Source: CAD feature listing. Evaluate the final solid. Frame: model axes, mm. A direction names the side the tool comes from. Give positions to 0.01 mm unless a question says otherwise; leave off trailing zeros. Write each loop counter-clockwise with the first axis right and the second up, starting at its lowest first coordinate (ties: lowest second). Pieces come first, ordered by that corner, then holes. Notation, with made-up numbers: (79.25, -14.75) -> (112.25, -14.75) arc R15 cw to (112.25, 9.25) -> close; hole circle Ø5 at (47, -24). An arc over 180 degrees is marked (long way). Answer as a JSON object with one key per item and string values. Group by question number.
Item 1: Section query A-A on z = 31. Return the cut outline in (x, y), plus the area to 3 significant figures.
Item 2: Pull-direction query (Y, two-part tool) for faces 1 (the face through (0, 30, 2)), 2 (the face through (0, 0, -19)), 3 (the face through (0, -30, 2)), 4 (the face through (26.438, 24.252, 1.726)); classes: pulls with the +Y half, pulls with the -Y half, needs draft (parallel to the pull), parting line crosses it, or undercut.
Item 3: Access query for faces 5 (the face through (0, -3, -13)), 6 (the face through (-23, -23, 3.5)), 7 (the face through (-1.615, 3.105, -9.367)), 8 (the face through (23, 23, 3.5)), 9 (the face through (-23, 23, 3.5)). Directions: +Z, -Z, +X, -X, +Y, -Y. A direction counts if a zero-diameter tool reaches every point of the face in a straight line with its end or side. Return the directions, or none.
Item 4: First-contact query: pin 1 Ø4 at (x, z) = (-1, -13.5) entering from -Y; pin 2 Ø1 at (x, z) = (0.5, -7) entering from +Y; pin 3 Ø3.5 at (x, y) = (25, 25) entering from -Z. Flat tips, straight axial feed; report the tip coordinate or a pass-through.
Item 5: Ray query, probe 1 along X at (y, z) = (25, 2); probe 2 along Z at (x, y) = (-7, -7.5). Return the intervals inside material, ascending. Write a range as from..to.
Autodesk Inventor part; units mm, degrees
ref_plane "YZ Plane" through (0, 0, 0) normal (1, 0, 0) x (0, 1, 0)
ref_plane "XZ Plane" through (0, 0, 0) normal (0, 1, 0) x (-1, 0, 0)
ref_plane "XY Plane" through (0, 0, 0) normal (0, 0, 1) x (1, 0, 0)
sketch "Esquisse1" plane through (0, 0, 0) normal (0, 0, 1) x (1, 0, 0)
  line L0 (-25.5, -30) -> (25.5, -30)
  line L1 (30, -25.5) -> (30, 25.5)
  line L2 (25.5, 30) -> (-25.5, 30)
  line L3 (-30, 25.5) -> (-30, -25.5)
  line L4 (-30, -30) -> (30, 30) construction
  line L5 (30, -30) -> (-30, 30) construction
  arc A0 (-30, -25.5) -> (-25.5, -30) centre (-25.5, -25.5) ccw
  arc A1 (25.5, -30) -> (30, -25.5) centre (25.5, -25.5) ccw
  arc A2 (30, 25.5) -> (25.5, 30) centre (25.5, 25.5) ccw
  arc A3 (-25.5, 30) -> (-30, 25.5) centre (-25.5, 25.5) ccw
  point P0 (0, 0)
  dimension "d0" = 60
  dimension "d1" = 60
  dimension "d2" = 4.5
extrude "Embase" add sketch "Esquisse1" along normal blind 3.5
sketch "Esquisse3" plane through (0, 0, 3.5) normal (0, 0, 1) x (1, 0, 0)
  point P0 (0, 0)
  point P1 (-25, -25)
  point P2 (-25, 25)
  point P3 (25, 25)
  point P4 (25, -25)
  dimension "Entraxe_moteur" = 50
  dimension "d8" = 50
  dimension "d9" = 25
  dimension "d10" = 25
hole "Perçage1" at (-25, -25, 3.5) at (-25, 25, 3.5) at (25, 25, 3.5) at (25, -25, 3.5) direction (0, 0, -1) diameter 3.242 end through all
sketch "Esquisse2" plane through (0, 0, 3.5) normal (0, 0, 1) x (1, 0, 0)
  circle A0 centre (0, 0) radius 30
  line L0 (-30, 25.5) -> (-30, -25.5)
extrude "Extrusion2" add sketch "Esquisse2" along normal blind 59
fillet "Congé1" radius 3 1 edges at (-30, 0, 62.5)
sketch "Esquisse4" plane through (0, 0, 0) normal (0, 0, -1) x (-1, 0, 0)
  circle A0 centre (0, 0) radius 3.5
  dimension "d19" = 7
extrude "Extrusion3" add sketch "Esquisse4" along normal blind 19
sketch "Esquisse5" plane through (0, 0, -19) normal (0, 0, -1) x (-1, 0, 0)
  line L0 (-1.8028, -3) -> (1.8028, -3)
  circle A0 centre (0, 0) radius 3.5
  dimension "d22" = 6.5
extrude "Extrusion4" cut sketch "Esquisse5" against normal blind 15 contours L0 A0 picked at (0.3722, -3.1057)
sketch "Esquisse6" plane through (-1.8028, -3, -19) normal (0, -1, 0) x (1, 0, 0)
  line L0 (3.6056, 0) -> (0, 0)
  point P0 (1.8028, 19)
  point P1 (1.8028, 8)
  point P2 (1.8028, 0)
  dimension "d25" = 8
hole "Perçage2" at (0, -3, -11) direction (0, 1, 0) diameter 3.4 end through all
properties part number "Moteur" material "Acier inoxydable"
Worked answers:
{
 "1": {"outline": "circle Ø60 at (0, 0)", "area": "2,830 mm^2"},
 "2": {"face 1": "pulls with the +Y half", "face 2": "needs draft", "face 3": "pulls with the -Y half", "face 4": "undercut"},
 "3": {"face 5": "-Z, +X, -X, -Y", "face 6": "+Z, -X, -Y", "face 7": "-Z", "face 8": "+Z, +X, +Y", "face 9": "+Z, -X, +Y"},
 "4": {"pin 1": "y = -3", "pin 2": "y = 3.5", "pin 3": "z = 0"},
 "5": {"probe 1": "-30..-26.62, -23.38..23.38, 26.62..30", "probe 2": "0..62.5"}
}
